Design review of the part built by this model. Coordinates are the model's own, in mm. A direction names the side the tool comes from. Give positions to 0.01 mm unless a question says otherwise; leave off trailing zeros. Loops run counter-clockwise (first coordinate to the right, second up) from the corner with the lowest first, then second, coordinate; pieces in that order, holes last. Notation, with made-up numbers: (65.25, 32.5) - (110.25, 32.5) arc R11 ccw to (110.25, 44.5) - close; hole circle Ø5 at (38, 39.5). An arc over 180 degrees is marked (long way). Write each question's results on one line, items separated by ' | '.
```python
from build123d import *

# Parameters (mm, degrees)
F7_DEPTH = 1


with BuildPart() as f2:
    # F0 (on Top) → F2 (revolve)
    with BuildSketch(Plane.XY):
        Polygon((20.4473696649, 3.5921053495), (20.4473696649, 0), (50.5868457019, 0), (50.5868457019, 2.7842106991), (49.9868457019, 2.7842106991), (49.9868457019, 0.6), (21.0473696649, 0.6), (21.0473696649, 4.1921053495), (16.9026321679, 4.1921053495), (16.9026321679, 8.0605266564), (12.1578937396, 8.0605266564), (12.1578937396, 7.4605266564), (16.3026321679, 7.4605266564), (16.3026321679, 3.5921053495), align=None)
    revolve(axis=Axis((0, 5.4080549162, 0), (0, -1, 0)))


with BuildPart() as f5:
    # F4 (on Front) → F5 (revolve)
    with BuildSketch(Plane.XZ):
        with BuildLine():
            Line((-62.6527036447, -1.87835907), (-52, 0))
            Line((-52, 0), (0, 0))
            Line((0, 0), (0, 1))
            Line((0, 1), (-52.0874886635, 1))
            Line((-52.0874886635, 1), (-62.8263518223, -0.893551317))
            ThreePointArc((-62.8263518223, -0.893551317), (-63.6427876097, -0.6747880071), (-64, 0.091256436))
            Line((-64, 0.091256436), (-64, 4.7077492508))
            Line((-64, 4.7077492508), (-65, 4.7077492508))
            Line((-65, 4.7077492508), (-65, 0.091256436))
            ThreePointArc((-65, 0.091256436), (-64.2855752194, -1.4408324503), (-62.6527036447, -1.87835907))
        make_face()
    revolve(axis=Axis((0, 0, -2.1538473566), (0, 0, -1)))

    # F6 (on face) → F7 (cut)
    with BuildSketch(Plane(origin=(0, 0, 0), x_dir=(1, 0, 0), z_dir=(0, 0, -1))):
        with BuildLine():
            ThreePointArc((-4, 45.6946386352), (-7.5, 49.1946386352), (-11, 45.6946386352))
            Line((-11, 45.6946386352), (-11, 7.5))
            ThreePointArc((-11, 7.5), (-7.5, 4), (-4, 7.5))
            Line((-4, 7.5), (-4, 45.6946386352))
        make_face()
        with BuildLine():
            ThreePointArc((-19, 39.1535439009), (-22.5, 42.6535439009), (-26, 39.1535439009))
            Line((-26, 39.1535439009), (-26, 7.5))
            ThreePointArc((-26, 7.5), (-22.5, 4), (-19, 7.5))
            Line((-19, 7.5), (-19, 39.1535439009))
        make_face()
        with BuildLine():
            ThreePointArc((-34, 22.9782505862), (-37.5, 26.4782505862), (-41, 22.9782505862))
            Line((-41, 22.9782505862), (-41, 7.5))
            ThreePointArc((-41, 7.5), (-37.5, 4), (-34, 7.5))
            Line((-34, 7.5), (-34, 22.9782505862))
        make_face()
        with BuildLine():
            ThreePointArc((-45.6946386352, -4), (-49.1946386352, -7.5), (-45.6946386352, -11))
            Line((-45.6946386352, -11), (-7.5, -11))
            ThreePointArc((-7.5, -11), (-4, -7.5), (-7.5, -4))
            Line((-7.5, -4), (-45.6946386352, -4))
        make_face()
        with BuildLine():
            Line((-7.5, -19), (-39.1535439009, -19))
            ThreePointArc((-39.1535439009, -19), (-42.6535439009, -22.5), (-39.1535439009, -26))
            Line((-39.1535439009, -26), (-7.5, -26))
            ThreePointArc((-7.5, -26), (-4, -22.5), (-7.5, -19))
        make_face()
        with BuildLine():
            Line((-7.5, -34), (-22.9782505862, -34))
            ThreePointArc((-22.9782505862, -34), (-26.4782505862, -37.5), (-22.9782505862, -41))
            Line((-22.9782505862, -41), (-7.5, -41))
            ThreePointArc((-7.5, -41), (-4, -37.5), (-7.5, -34))
        make_face()
        with BuildLine():
            ThreePointArc((4, -45.6946386352), (7.5, -49.1946386352), (11, -45.6946386352))
            Line((11, -45.6946386352), (11, -7.5))
            ThreePointArc((11, -7.5), (7.5, -4), (4, -7.5))
            Line((4, -7.5), (4, -45.6946386352))
        make_face()
        with BuildLine():
            Line((19, -7.5), (19, -39.1535439009))
            ThreePointArc((19, -39.1535439009), (22.5, -42.6535439009), (26, -39.1535439009))
            Line((26, -39.1535439009), (26, -7.5))
            ThreePointArc((26, -7.5), (22.5, -4), (19, -7.5))
        make_face()
        with BuildLine():
            Line((34, -7.5), (34, -22.9782505862))
            ThreePointArc((34, -22.9782505862), (37.5, -26.4782505862), (41, -22.9782505862))
            Line((41, -22.9782505862), (41, -7.5))
            ThreePointArc((41, -7.5), (37.5, -4), (34, -7.5))
        make_face()
        with BuildLine():
            ThreePointArc((45.6946386352, 4), (49.1946386352, 7.5), (45.6946386352, 11))
            Line((45.6946386352, 11), (7.5, 11))
            ThreePointArc((7.5, 11), (4, 7.5), (7.5, 4))
            Line((7.5, 4), (45.6946386352, 4))
        make_face()
        with BuildLine():
            Line((7.5, 19), (39.1535439009, 19))
            ThreePointArc((39.1535439009, 19), (42.6535439009, 22.5), (39.1535439009, 26))
            Line((39.1535439009, 26), (7.5, 26))
            ThreePointArc((7.5, 26), (4, 22.5), (7.5, 19))
        make_face()
        with BuildLine():
            Line((7.5, 34), (22.9782505862, 34))
            ThreePointArc((22.9782505862, 34), (26.4782505862, 37.5), (22.9782505862, 41))
            Line((22.9782505862, 41), (7.5, 41))
            ThreePointArc((7.5, 41), (4, 37.5), (7.5, 34))
        make_face()
    extrude(amount=-F7_DEPTH, mode=Mode.SUBTRACT)


solid = f5.part
```
Item 1: Wall thickness on probe 1 along Z at (x, y) = (45.5, 15.5); probe 2 along Y at (x, z) = (0, 1.3); probe 3 along Y at (x, z) = (-16, 3.5): over which ranges is each line inside the solid? List them lowest first.
Output values:
probe 1: z = 0 to 1 | probe 2: y = -65 to -64, 64 to 65 | probe 3: y = -63 to -61.97, 61.97 to 63
Item 2: Tool access review of faces 1 (the face through (11.38, -51.27, -0.09)), 2 (the face through (37.423, 26.477, 0.493)): name each direction out of +Z, -Z, +X, -X, +Y, -Y from which nothing blocks a thin tool from reaching the whole face with its end or side.
Output values:
face 1: -Z | face 2: +Z, -Z
Item 3: We need section B-B on z = 2.25. Give the boundary of the cut face in (x, y), then the cut area to 3 significant figures.
Output values:
outline: circle Ø130 at (0, 0); hole circle Ø128 at (0, 0) | area: 405 mm²
Item 4: Clearance check with flat-ended pins moving along their axes: P1, Ø2, axis at x = -38.5, z = 2.5, coming from the +Y side; P2, Ø0.8, axis at x = 28, z = 0.5, coming from the -Y side; P3, Ø0.8, axis at x = -25.5, z = 0.5, coming from the -Y side. State where each tip first meets the part, or that it passes through.
Output values:
P1: stops at y = 53.09 | P2: stops at y = -58.85 | P3: stops at y = -59.96
Item 5: We need section A-A on y = 0. Give the boundary of the cut face in (x, z), then the cut area to 3 significant figures.
Output values:
outline: (-65, 0.09) arc R2 ccw to (-62.65, -1.88) - (-52, 0) - (52, 0) - (62.65, -1.88) arc R2 ccw to (65, 0.09) - (65, 4.71) - (64, 4.71) - (64, 0.09) arc R1 cw to (62.83, -0.89) - (52.09, 1) - (-52.09, 1) - (-62.83, -0.89) arc R1 cw to (-64, 0.09) - (-64, 4.71) - (-65, 4.71) - close | area: 140 mm²
Item 6: We need section C-C on x = -37.5. Give the number of separate pieces and of enclosed holes in the cut face, then the cut area to 3 significant figures.
Output values:
separate pieces: 4 | enclosed holes: 0 | area: 82.4 mm²
Item 7: Draft analysis for pull direction Y (two halves, no side actions). For faces 3 (the face through (48, -43, 4.708)), 4 (the face through (-62, 19.52, 2.37)), 5 (the face through (22.423, 42.653, 0.493)), 6 (the face through (-22.423, -42.653, 0.493)), state which applies: +Y half, -Y half, draft (parallel to the pull), parting line (faces both ways), or undercut.
Output values:
face 3: draft | face 4: parting line | face 5: undercut | face 6: undercut
